from build123d import *

# Parameters (mm, degrees)
SKETCH1_W               = 200
SKETCH1_H               = 50
BOSS_EXTRUDE1_DEPTH     = 1.5
SKETCH3_R               = 5
CUT_EXTRUDE2_DEPTH      = 108.976849371
CUT_EXTRUDE3_DEPTH      = 108.976849371
CUT_EXTRUDE3_DEPTH_BACK = 108.976849371
SKETCH4_R               = 1.5
CUT_EXTRUDE4_DEPTH      = 108.976849371
CUT_EXTRUDE4_DEPTH_BACK = 108.976849371
SKETCH5_W               = 34
SKETCH5_H               = 26
CUT_EXTRUDE5_DEPTH      = 108.976849371
CUT_EXTRUDE5_DEPTH_BACK = 108.976849371
SKETCH6_W               = 25
SKETCH6_H               = 5


with BuildPart() as part:
    # Sketch1 → Boss-Extrude1 (new, symmetric)
    with BuildSketch(Plane(origin=(0, 0, 0), x_dir=(1, 0, 0), z_dir=(0, 1, 0))):
        with Locations((5, 0)):
            Rectangle(SKETCH1_W, SKETCH1_H)
    extrude(amount=BOSS_EXTRUDE1_DEPTH, both=True)

    # Sketch3 → Cut-Extrude2 (cut, through all)
    with BuildSketch(Plane(origin=(0, 1.5, 0), x_dir=(1, 0, 0), z_dir=(0, 1, 0))):
        with Locations(Location((12, 0, 0), (0, 0, 270))):
            Circle(SKETCH3_R)
    extrude(amount=-CUT_EXTRUDE2_DEPTH, mode=Mode.SUBTRACT)

    # Sketch4 → Cut-Extrude3 (cut, two sides: drawn at the far end of the back side and taken through both)
    with BuildSketch(Plane(origin=(0, 1.5, 0), x_dir=(1, 0, 0), z_dir=(0, 1, 0)).offset(-CUT_EXTRUDE3_DEPTH_BACK)):
        with Locations(Location((65, 3.75, 0), (0, 0, 270))):
            Circle(SKETCH4_R)
        with Locations(Location((95, 3.75, 0), (0, 0, 270))):
            Circle(SKETCH4_R)
        with Locations(Location((95, -3.75, 0), (0, 0, 90))):
            Circle(SKETCH4_R)
        with Locations(Location((65, -3.75, 0), (0, 0, 90))):
            Circle(SKETCH4_R)
    extrude(amount=CUT_EXTRUDE3_DEPTH + CUT_EXTRUDE3_DEPTH_BACK, mode=Mode.SUBTRACT)

    # Sketch5 → Cut-Extrude4 (cut, two sides: drawn at the far end of the back side and taken through both)
    with BuildSketch(Plane(origin=(0, 1.5, 0), x_dir=(1, 0, 0), z_dir=(0, 1, 0)).offset(-CUT_EXTRUDE4_DEPTH_BACK)):
        with Locations((43, -1)):
            Rectangle(SKETCH5_W, SKETCH5_H)
    extrude(amount=CUT_EXTRUDE4_DEPTH + CUT_EXTRUDE4_DEPTH_BACK, mode=Mode.SUBTRACT)

    # Sketch6 → Cut-Extrude5 (cut, two sides: drawn at the far end of the back side and taken through both)
    with BuildSketch(Plane(origin=(0, 1.5, 0), x_dir=(1, 0, 0), z_dir=(0, 1, 0)).offset(-CUT_EXTRUDE5_DEPTH_BACK)):
        with Locations((43, 14.5)):
            Rectangle(SKETCH6_W, SKETCH6_H)
    extrude(amount=CUT_EXTRUDE5_DEPTH + CUT_EXTRUDE5_DEPTH_BACK, mode=Mode.SUBTRACT)


solid = part.part
Geometry: final body of the model. Coordinates: model frame, mm. Give positions to 0.01 mm unless a question says otherwise; leave off trailing zeros. Write each loop counter-clockwise with the first axis right and the second up, starting at its lowest first coordinate (ties: lowest second). Pieces come first, ordered by that corner, then holes. Notation, with made-up numbers: (24, -32.5) -> (32, -32.5) arc R13 cw to (32, -22.5) -> close; hole circle Ø10 at (77.5, 50.25). An arc over 180 degrees is marked (long way). Answer as a JSON object with one key per item and string values.
1. Cut plane C-C on z = 0. Output: boundary loops of the cut face in (x, y), and give its area (3 significant figures).
Ans:
{"outline": "(-95, -1.5) -> (7, -1.5) -> (7, 1.5) -> (-95, 1.5) -> close; (17, -1.5) -> (26, -1.5) -> (26, 1.5) -> (17, 1.5) -> close; (60, -1.5) -> (105, -1.5) -> (105, 1.5) -> (60, 1.5) -> close", "area": "468 mm^2"}
2. Cut plane D-D on y = -0.05. Output: boundary loops of the cut face in (x, z).
Ans:
{"outline": "(-95, -25) -> (105, -25) -> (105, 25) -> (-95, 25) -> close; hole circle Ø10 at (12, 0); hole (26, -12) -> (30.5, -12) -> (30.5, -17) -> (55.5, -17) -> (55.5, -12) -> (60, -12) -> (60, 14) -> (26, 14) -> close; hole circle Ø3 at (65, -3.75); hole circle Ø3 at (65, 3.75); hole circle Ø3 at (95, -3.75); hole circle Ø3 at (95, 3.75)"}
3. Cut plane B-B on x = 12. Output: boundary loops of the cut face in (y, z), and give its area (3 significant figures).
Ans:
{"outline": "(-1.5, -25) -> (1.5, -25) -> (1.5, -5) -> (-1.5, -5) -> close; (-1.5, 5) -> (1.5, 5) -> (1.5, 25) -> (-1.5, 25) -> close", "area": "120 mm^2"}
4. Cut plane A-A on z = 11. Output: boundary loops of the cut face in (x, y).
Ans:
{"outline": "(-95, -1.5) -> (26, -1.5) -> (26, 1.5) -> (-95, 1.5) -> close; (60, -1.5) -> (105, -1.5) -> (105, 1.5) -> (60, 1.5) -> close"}
5. Ray query, probe 1 along X at (y, z) = (-0.2, 0); probe 2 along X at (y, z) = (0.8, 7.5); probe 3 along Z at (x, y) = (45, -0.75). Return the intervals inside material, ascending. Write a range as from..to.
Ans:
{"probe 1": "x = -95..7, 17..26, 60..105", "probe 2": "x = -95..26, 60..105", "probe 3": "z = -25..-17, 14..25"}
6. Mould query, pull axis Z, two halves, no side actions, for faces 1 (the flat face through (4, -1.5, 0)), 2 (the cylindrical face through (16.957, 0.021, -0.651)). Classes: pulls with the +Z half, pulls with the -Z half, needs draft (parallel to the pull), parting line crosses it, or undercut.
Ans:
{"face 1": "needs draft", "face 2": "undercut"}
